Source: three-view drawing plus pictorial views. Frame: mm from the lowest corner of the part. A direction names the side the tool comes from. Give positions to 0.01 mm unless a question says otherwise; leave off trailing zeros. Loops run counter-clockwise (first coordinate to the right, second up) from the corner with the lowest first, then second, coordinate; pieces in that order, holes last.
1. Material intervals for line 1 along Y through (x, z) = (6, 1.4); line 2 along Y through (x, z) = (18.5, 3.6); line 3 along Z through (x, y) = (13, 4.5), sorted ascending.
2. Section A-A, the plane y = 4.5. Output: boundary loops of the cut face in (x, z).
3. Section D-D, the plane x = 14.5. Output: boundary loops of the cut face in (y, z), then the cut area to 3 significant figures.
4. Access query for the marked faces 1 and 2. Directions: +Z, -Z, +X, -X, +Y, -Y. A direction counts if a zero-diameter tool reaches every point of the face in a straight line with its end or side. Return the directions, or none.
5. Section C-C, the plane z = 2.55. Output: boundary loops of the cut face in (x, y), then the cut area to 3 significant figures.
6. First-contact query: P1, Ø1.5, axis at x = 7.5, y = 4, coming from the -Z side; P2, Ø1.6, axis at y = 4, z = 3.5, coming from the -X side; P3, Ø3, axis at x = 14, y = 5, coming from the +Z side. Flat tips, straight axial feed; report the tip coordinate or a pass-through.
7. Section B-B, the plane x = 7.5. Output: boundary loops of the cut face in (y, z), then the cut area to 3 significant figures.
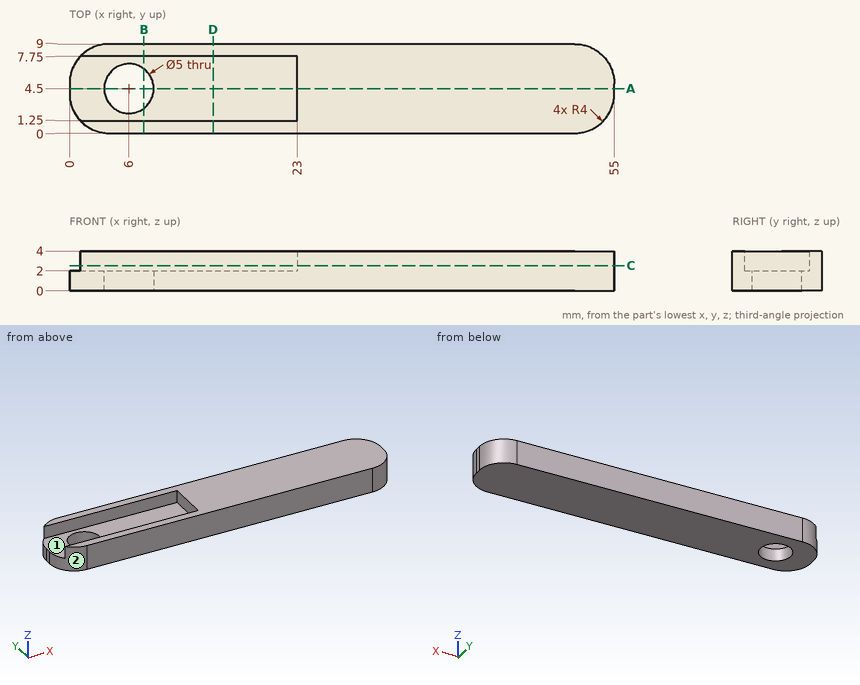
Answers below:
1. line 1: y = 0 to 2, 7 to 9
1. line 2: y = 0 to 1.25, 7.75 to 9
1. line 3: z = 0 to 2
2. outline: (0, 0) - (3.5, 0) - (3.5, 2) - (0, 2) - close; (8.5, 0) - (55, 0) - (55, 4) - (23, 4) - (23, 2) - (8.5, 2) - close
3. outline: (0, 0) - (9, 0) - (9, 4) - (7.75, 4) - (7.75, 2) - (1.25, 2) - (1.25, 4) - (0, 4) - close
3. area: 23.0 mm2
4. face 1: +Z, -X
4. face 2: +Z, -Z, -X, -Y
5. outline: (1.1, 1.25) arc R4 ccw to (4, 0) - (51, 0) arc R4 ccw to (55, 4) - (55, 5) arc R4 ccw to (51, 9) - (4, 9) arc R4 ccw to (1.1, 7.75) - (23, 7.75) - (23, 1.25) - close
5. area: 334 mm2
6. P1: passes through
6. P2: stops at x = 23
6. P3: stops at z = 2
7. outline: (0, 0) - (2.5, 0) - (2.5, 2) - (1.25, 2) - (1.25, 4) - (0, 4) - close; (6.5, 0) - (9, 0) - (9, 4) - (7.75, 4) - (7.75, 2) - (6.5, 2) - close
7. area: 15.0 mm2
